```python
from build123d import *

# Parameters (mm, degrees)
F0_W        = 71.6
F0_H        = 14.35
F1_DEPTH    = 32.56
F2_T1_DEPTH = 69.06


# Not quite as in the source:
# - a fillet or chamfer that OpenCascade refuses, or shapes differently, is made with other operations: its cross-section is extruded or revolved along the edge and cut away or added


with BuildPart() as f1:
    # F0 (on Front) → F1 (new body)
    with BuildSketch(Plane.XZ):
        Rectangle(F0_W, F0_H)
    extrude(amount=F1_DEPTH)

    # F2: fillet of radius 7.3 on 2 edges, made by hand

    # F2_s2 → F2_t1 (cut)
    with BuildSketch(Plane.XZ.offset(-18.25)):
        with BuildLine():
            ThreePointArc((-28.5, 7.175), (-33.6618795027, 5.0368795027), (-35.8, -0.125))
            Line((-35.8, -0.125), (-35.8, 7.175))
            Line((-35.8, 7.175), (-28.5, 7.175))
        make_face()
        with BuildLine():
            ThreePointArc((-35.8, 0.125), (-33.6618795027, -5.0368795027), (-28.5, -7.175))
            Line((-28.5, -7.175), (-35.8, -7.175))
            Line((-35.8, -7.175), (-35.8, 0.125))
        make_face()
    extrude(amount=F2_T1_DEPTH, mode=Mode.SUBTRACT)


solid = f1.part
```
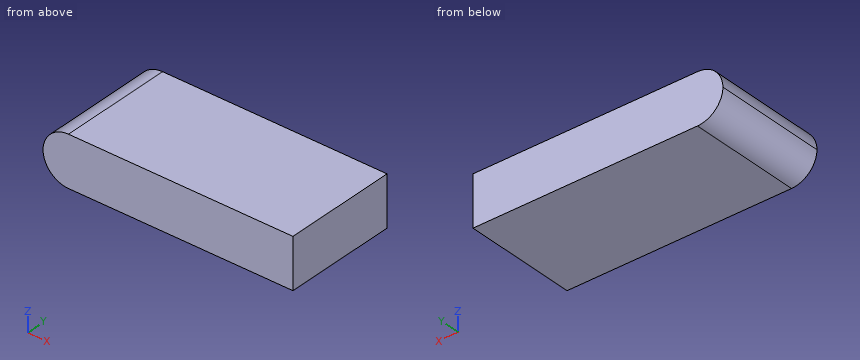
Source: CAD feature listing. Evaluate the final solid. Frame: model axes, mm. Coordinates: 2 decimals unless noted, no trailing zeros. Write each loop counter-clockwise with the first axis right and the second up, starting at its lowest first coordinate (ties: lowest second). Pieces come first, ordered by that corner, then holes. Notation, with made-up numbers: (-32.75, 69) - (19.25, 69) arc R8 ccw to (19.25, 79) - close; hole circle Ø1 at (24, -11.75). An arc over 180 degrees is marked (long way). Answer as a JSON object with one key per item and string values.
Q1. Material intervals for line 1 (X direction, y = -25.5, z = 0.25); line 2 (X direction, y = -6, z = -4), sorted ascending. Write a range as [from, to].
Ans:
{"line 1": "x = [-35.79, 35.8]", "line 2": "x = [-34.52, 35.8]"}
Q2. Section query B-B, the plane z = -4.75. Output: boundary loops of the cut face in (x, y), plus the area to 3 significant figures.
Ans:
{"outline": "(-33.93, -32.56) - (35.8, -32.56) - (35.8, 0) - (-33.93, 0) - close", "area": "2,270 mm2"}
Q3. Section query A-A, the plane y = -30.5. Output: boundary loops of the cut face in (x, z) (3 decimals).
Ans:
{"outline": "(-35.799, 0) arc R7.3 ccw to (-28.5, -7.175) - (35.8, -7.175) - (35.8, 7.175) - (-28.5, 7.175) arc R7.3 ccw to start"}
Q4. Section query C-C, the plane z = 6. Output: boundary loops of the cut face in (x, y).
Ans:
{"outline": "(-32.47, -32.56) - (35.8, -32.56) - (35.8, 0) - (-32.47, 0) - close"}
